Design review of the part built by this model. Coordinates are the model's own, in mm. Face numbers are marked on the shaded views. A direction names the side the tool comes from. Give positions to 0.01 mm unless a question says otherwise; leave off trailing zeros. Order: outer loops, then holes, each group sorted by start corner. A loop starts at its lowest first (then second) coordinate and runs counter-clockwise, first axis right, second up. Notation, with made-up numbers: (18.5, -27) -> (55.5, -27) arc R10 cw to (55.5, -17) -> close; hole circle Ø2 at (-2.5, 10.5). An arc over 180 degrees is marked (long way). One line per item, written item: value.
from build123d import *

# Parameters (mm, degrees)
SKETCH002_W   = 44.6
SKETCH002_H   = 24.4
SKETCH002_W_2 = 40.6
SKETCH002_H_2 = 20.4
PAD001_DEPTH  = 12
BOX_W         = 44.2
BOX_H         = 24.2
BOX_DEPTH     = 2
PAD_DEPTH     = 2.5
SKETCH003_W   = 15
SKETCH003_H   = 25
PAD002_DEPTH  = 10
PAD003_DEPTH  = 2


with BuildPart() as part:
    # Sketch002 → Pad001 (new body)
    with BuildSketch(Plane.XY):
        with Locations((20.3, 10.2)):
            Rectangle(SKETCH002_W, SKETCH002_H)
        with Locations((20.3, 10.2)):
            Rectangle(SKETCH002_W_2, SKETCH002_H_2, mode=Mode.SUBTRACT)
    extrude(amount=PAD001_DEPTH)

    # Box → Box (join)
    with BuildSketch(Plane(origin=(-2, -2, 10), x_dir=(1, 0, 0), z_dir=(0, 0, 1))):
        with Locations((22.1, 12.1)):
            Rectangle(BOX_W, BOX_H)
    extrude(amount=BOX_DEPTH)

    # Sketch → Pad (join, symmetric)
    with BuildSketch(Plane.YZ.offset(5.5)):
        Polygon((-25, -10), (-2, -40), (0, -40), (0, -10), (0, 12), (-5, 12), (-5, -5), (-12.5, -15), (-20, -5), (-20, 12), (-25, 12), align=None)
    extrude(amount=PAD_DEPTH, both=True)

    # Sketch003 → Pad002 (join)
    with BuildSketch(Plane.XY.offset(12)):
        with Locations((5.5, -12.5)):
            Rectangle(SKETCH003_W, SKETCH003_H)
        with BuildLine():
            Line((3, -5), (3, -20))
            ThreePointArc((3, -20), (5.5, -22.5), (8, -20))
            Line((8, -20), (8, -5))
            ThreePointArc((8, -5), (5.5, -2.5), (3, -5))
        make_face(mode=Mode.SUBTRACT)
    extrude(amount=-PAD002_DEPTH)

    # Sketch004 → Pad003 (join)
    with BuildSketch(Plane.XZ):
        Polygon((-2, 0), (-2, -40), (8, -40), (42.6, 0), align=None)
    extrude(amount=PAD003_DEPTH)


solid = part.part
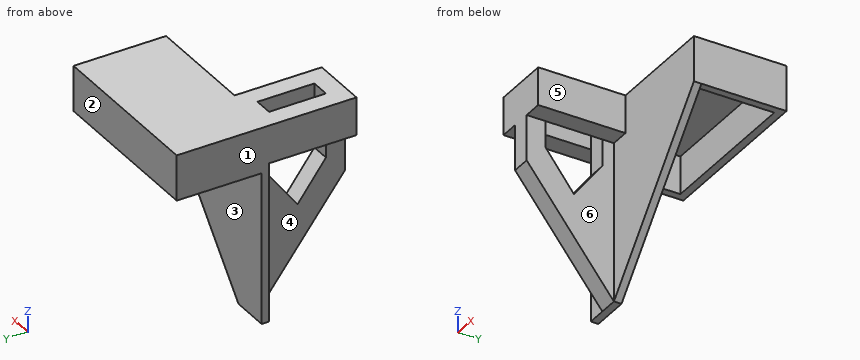
Item 1: Add section C-C on y = 19.5. Give the boundary of the cut face in (x, z), plus the area to 3 significant figures.
Returned:
outline: (-2, 0) -> (0, 0) -> (0, 10) -> (40.6, 10) -> (40.6, 0) -> (42.6, 0) -> (42.6, 12) -> (-2, 12) -> close
area: 129 mm²
Item 2: Add section A-A on z = -6. Give the boundary of the cut face in (x, y).
Returned:
outline: (-2, -2) -> (3, -2) -> (3, -5.75) -> (8, -5.75) -> (8, -2) -> (37.41, -2) -> (37.41, 0) -> (-2, 0) -> close; (3, -25) -> (8, -25) -> (8, -19.25) -> (3, -19.25) -> close
Item 3: Add section B-B on x = 1. Give the boundary of the cut face in (y, z).
Returned:
outline: (-25, 2) -> (-2, 2) -> (-2, -40) -> (0, -40) -> (0, 10) -> (20.4, 10) -> (20.4, 0) -> (22.4, 0) -> (22.4, 12) -> (-25, 12) -> close
Item 4: Draft analysis for pull direction Y (two halves, no side actions). For the marked faces 1, 2 and 3, state which applies: pulls with the +Y half, pulls with the -Y half, needs draft (parallel to the pull), parting line crosses it, or undercut.
Returned:
face 1: needs draft
face 2: pulls with the +Y half
face 3: undercut
Item 5: Add section D-D on z = 6. Give the boundary of the cut face in (x, y), plus the area to 3 significant figures.
Returned:
outline: (-2, -25) -> (13, -25) -> (13, -2) -> (42.6, -2) -> (42.6, 22.4) -> (-2, 22.4) -> close; hole (0, 0) -> (40.6, 0) -> (40.6, 20.4) -> (0, 20.4) -> close; hole (3, -20) -> (8, -20) -> (8, -5) -> (3, -5) -> close
area: 530 mm²
Item 6: Machinability: for the marked faces 4, 5 and 6, which of the approach directions +Z, -Z, +X, -X, +Y, -Y give a long, thin tool a straight path to every point of the face, cutting with its end or side? Answer none if there is none.
Returned:
face 4: -Z, -X, -Y
face 5: +Z, -Z, +X, -Y
face 6: -Z, +X, -Y
Item 7: Clearance check with flat-ended pins moving along their axes: P1, Ø2, axis at x = 11.5, z = -29.5, coming from the +Y side; P2, Ø4, axis at x = -0.5, z = -23.5, coming from the -Y side; P3, Ø7, axis at y = -8, z = -17, coming from the -X side; P4, Ø13.5, axis at x = 9.5, z = -4.5, coming from the +Y side. State where each tip first meets the part, or that it passes through.
Returned:
P1: y = 0
P2: y = -2
P3: x = 3
P4: y = 22.4
Item 8: To check wall thickness, follow line 1 along X through (y, z) = (-8, 3.5); line 2 along Z through (x, y) = (10.5, -13.5); line 3 along Z through (x, y) = (26, 7). State the ranges of each line that lie inside material, in increasing order. Write a range as from..to.
Returned:
line 1: -2..3, 8..13
line 2: 2..12
line 3: 10..12
